Geometry: final body of the model. Coordinates: model frame, mm. A direction names the side the tool comes from. Round coordinates to 2 decimals unless told otherwise and drop trailing zeros. Write each loop counter-clockwise with the first axis right and the second up, starting at its lowest first coordinate (ties: lowest second). Pieces come first, ordered by that corner, then holes. Notation, with made-up numbers: M 50,25 L 102,25 A14 cw 102,44 Z; hole C -6,85.25 d7. An arc over 180 degrees is marked long. Answer as CSV lines item,"result". Start each with the question number.
Q1. Mould query, pull axis Z, two halves, no side actions, for faces 4 (the flat face through (-6, 21, 17)), 5 (the flat face through (0, 0, 44)), 6 (the cylindrical face through (0, 5, 40)). Classes: pulls with the +Z half, pulls with the -Z half, needs draft (parallel to the pull), parting line crosses it, or undercut.
Q2. Section query C-C on z = 38. Output: boundary loops of the cut face in (x, y), and give its area (3 significant figures).
Q3. Section query D-D on x = -17. Output: boundary loops of the cut face in (y, z).
Q4. Section query B-B on x = 0. Output: boundary loops of the cut face in (y, z), and give its area (3 significant figures).
Q5. Section query A-A on y = 16. Give the number of separate pieces and of enclosed holes in the cut face, and give its area (3 significant figures).
Q6. First-contact query: pin 1 (17.5 mm diameter, centred on y = 3, z = 39.5, fed in from -X); pin 2 (7 mm diameter, centred on x = 15, y = -2, fed in from +Z); pin 3 (2.5 mm diameter, centred on x = -8, z = 17, fed in from +Y); pin 4 (6 mm diameter, centred on y = 11, z = 31.5, fed in from +X). Flat tips, straight axial feed; report the tip coordinate or a pass-through.
Q7. Reachability of faces 1 (the flat face through (-10, 0, 36)), 2 (the flat face through (10, 0, 36)), 3 (the cylindrical face through (0.07, 0.29, 23.5)) from +Z, -Z, +X, -X, +Y, -Y: full face, straight path, thin tool, end or side. Return the list, or none.
Q8. Ray query, probe 1 along Y at (x, z) = (1, 38); probe 2 along X at (y, z) = (7, 25); probe 3 along X at (y, z) = (1.5, 36.5). Return the intervals inside material, ascending.
```python
from build123d import *

# Parameters (mm, degrees)
SKETCH_1_W          = 48
SKETCH_1_H          = 42
EXTRUDE_1_DEPTH     = 38
SKETCH_3_R          = 6
SKETCH_3_R_2        = 5.5
SKETCH_3_R_3        = 1.5
CUT_EXTRUDE_2_DEPTH = 62.514225997
SKETCH_9_W          = 14
SKETCH_9_H          = 10
CUT_EXTRUDE_6_DEPTH = 62.514225997
SKETCH_10_W         = 20
SKETCH_10_H         = 6
EXTRUDE_3_DEPTH     = 42
SKETCH_11_R         = 2
CUT_EXTRUDE_7_DEPTH = 60.439044407


with BuildPart() as part:
    # 草圖1 → 填料-伸長1 (new body)
    with BuildSketch(Plane.XY):
        Rectangle(SKETCH_1_W, SKETCH_1_H)
    extrude(amount=EXTRUDE_1_DEPTH)

    # 草圖3 → 除料-伸長2 (cut, through all)
    with BuildSketch(Plane(origin=(0, 21, 0), x_dir=(1, 0, 0), z_dir=(0, 1, 0))):
        with Locations(Location((17, -17, 0), (0, 0, 270))):
            Circle(SKETCH_3_R)
        with Locations(Location((-17, -17, 0), (0, 0, 270))):
            Circle(SKETCH_3_R)
        with Locations(Location((0, -17, 0), (0, 0, 270))):
            Circle(SKETCH_3_R_2)
        with Locations(Location((0, -25, 0), (0, 0, 270))):
            Circle(SKETCH_3_R_3)
        with Locations(Location((8, -17, 0), (0, 0, 270))):
            Circle(SKETCH_3_R_3)
        with Locations(Location((0, -9, 0), (0, 0, 270))):
            Circle(SKETCH_3_R_3)
        with Locations(Location((-8, -17, 0), (0, 0, 270))):
            Circle(SKETCH_3_R_3)
    extrude(amount=-CUT_EXTRUDE_2_DEPTH, mode=Mode.SUBTRACT)

    # 草圖9 → 除料-伸長6 (cut, through all)
    with BuildSketch(Plane(origin=(0, 21, 0), x_dir=(1, 0, 0), z_dir=(0, 1, 0))):
        with Locations((-17, -33)):
            Rectangle(SKETCH_9_W, SKETCH_9_H)
        with Locations((17, -33)):
            Rectangle(SKETCH_9_W, SKETCH_9_H)
    extrude(amount=-CUT_EXTRUDE_6_DEPTH, mode=Mode.SUBTRACT)

    # 草圖10 → 填料-伸長3 (add)
    with BuildSketch(Plane(origin=(0, 21, 0), x_dir=(1, 0, 0), z_dir=(0, 1, 0))):
        with Locations((0, -41)):
            Rectangle(SKETCH_10_W, SKETCH_10_H)
    extrude(amount=-EXTRUDE_3_DEPTH)

    # 草圖11 → 除料-伸長7 (cut, through all)
    with BuildSketch(Plane(origin=(10, 0, 0), x_dir=(0, 0, -1), z_dir=(1, 0, 0))):
        with Locations((-38, 16)):
            Circle(SKETCH_11_R)
        with Locations((-38, 5)):
            Circle(SKETCH_11_R)
        with Locations((-38, -5)):
            Circle(SKETCH_11_R)
        with Locations((-38, -16)):
            Circle(SKETCH_11_R)
    extrude(amount=-CUT_EXTRUDE_7_DEPTH, mode=Mode.SUBTRACT)


solid = part.part
```
Entries:
1,face 4,"needs draft"
1,face 5,"pulls with the +Z half"
1,face 6,"undercut"
2,outline,"M -10,-21 L 10,-21 L 10,-18 L -10,-18 Z; M -10,-14 L 10,-14 L 10,-7 L -10,-7 Z; M -10,-3 L 10,-3 L 10,3 L -10,3 Z; M -10,7 L 10,7 L 10,14 L -10,14 Z; M -10,18 L 10,18 L 10,21 L -10,21 Z"
2,area,"520 mm^2"
3,outline,"M -21,0 L 21,0 L 21,11 L -21,11 Z; M -21,23 L 21,23 L 21,28 L -21,28 Z"
4,outline,"M -21,0 L 21,0 L 21,7.5 L -21,7.5 Z; M -21,10.5 L 21,10.5 L 21,11.5 L -21,11.5 Z; M -21,22.5 L 21,22.5 L 21,23.5 L -21,23.5 Z; M -21,26.5 L 21,26.5 L 21,44 L -21,44 Z; hole C -16,38 d4; hole C -5,38 d4; hole C 5,38 d4; hole C 16,38 d4"
4,area,"1,080 mm^2"
5,separate pieces,"2"
5,enclosed holes,"7"
5,area,"1,230 mm^2"
6,pin 1,"stops at x = -10"
6,pin 2,"stops at z = 28"
6,pin 3,"passes through"
6,pin 4,"stops at x = 10"
7,face 1,"+Z, -X, +Y, -Y"
7,face 2,"+Z, +X, +Y, -Y"
7,face 3,"+Y, -Y"
8,probe 1,"y = -21 to -18, -14 to -7, -3 to 3, 7 to 14, 18 to 21"
8,probe 2,"x = -24 to -1.5, 1.5 to 24"
8,probe 3,"x = -10 to 10"
